CAD build for the part. Positions are in the model's coordinates, mm. A direction names the side the tool comes from. Give positions to 0.01 mm unless a question says otherwise; leave off trailing zeros. Write each loop counter-clockwise with the first axis right and the second up, starting at its lowest first coordinate (ties: lowest second). Pieces come first, ordered by that corner, then holes. Notation, with made-up numbers: (-5.75, 11.5) -> (39.25, 11.5) arc R33 ccw to (39.25, 47.5) -> close; hole circle Ø3 at (81.25, 41). An arc over 180 degrees is marked (long way). Answer as a JSON object with one key per item and string values.
```python
from build123d import *

# Parameters (mm, degrees)
SKICA2_W                 = 72.4
SKICA2_H                 = 47.7
P_IDAT_VYSUNUT_M1_DEPTH  = 1.2
SKICA3_W                 = 70
SKICA3_H                 = 46.5
P_IDAT_VYSUNUT_M2_DEPTH  = 1
SKICA4_W                 = 70
SKICA4_H                 = 7
P_IDAT_VYSUNUT_M3_DEPTH  = 7
ZKOSEN_2_SIZE            = 7
SKICA5_W                 = 15
SKICA5_H                 = 2
ODEBRAT_VYSUNUT_M1_DEPTH = 10
SKICA6_W                 = 15
SKICA6_H                 = 1.2
ODEBRAT_VYSUNUT_M2_DEPTH = 1


with BuildPart() as part:
    # Skica2 → Přidat vysunutím1 (new body)
    with BuildSketch(Plane(origin=(0, 0, 0), x_dir=(1, 0, 0), z_dir=(0, 1, 0))):
        with Locations((36.2, 23.85)):
            Rectangle(SKICA2_W, SKICA2_H)
    extrude(amount=P_IDAT_VYSUNUT_M1_DEPTH)

    # Skica3 → Přidat vysunutím2 (add)
    with BuildSketch(Plane(origin=(0, 1.2, 0), x_dir=(1, 0, 0), z_dir=(0, 1, 0))):
        with Locations((36.2, 24.45)):
            Rectangle(SKICA3_W, SKICA3_H)
    extrude(amount=P_IDAT_VYSUNUT_M2_DEPTH)

    # Skica4 → Přidat vysunutím3 (add)
    with BuildSketch(Plane(origin=(0, 2.2, 0), x_dir=(1, 0, 0), z_dir=(0, 1, 0))):
        with Locations((36.2, 44.2)):
            Rectangle(SKICA4_W, SKICA4_H)
    extrude(amount=P_IDAT_VYSUNUT_M3_DEPTH)

    # Zkosení2
    zkosen_2_edges = [part.edges().sort_by_distance(p)[0] for p in [
        (36.2, 9.2, -40.7),
    ]]
    chamfer(zkosen_2_edges, length=ZKOSEN_2_SIZE - 0.0001)  # a hair under: the kernel refuses the full size

    # Skica5 → Odebrat vysunutím1 (cut)
    with BuildSketch(Plane(origin=(0, 2.2, 0), x_dir=(1, 0, 0), z_dir=(0, 1, 0))):
        with Locations((36.2, 1)):
            Rectangle(SKICA5_W, SKICA5_H)
    extrude(amount=-ODEBRAT_VYSUNUT_M1_DEPTH, mode=Mode.SUBTRACT)

    # Skica6 → Odebrat vysunutím2 (cut)
    with BuildSketch(Plane(origin=(0, 2.2, 0), x_dir=(1, 0, 0), z_dir=(0, 1, 0))):
        with Locations((36.2, 2.6)):
            Rectangle(SKICA6_W, SKICA6_H)
    extrude(amount=-ODEBRAT_VYSUNUT_M2_DEPTH, mode=Mode.SUBTRACT)


solid = part.part
```
1) Pin check, flat tips, straight feed: pin 1 (0.5 mm diameter, centred on x = 13.5, y = 1.5, fed in from +Z); pin 2 (12 mm diameter, centred on x = 11, z = -35, fed in from +Y); pin 3 (1.1 mm diameter, centred on x = 39, y = 1.5, fed in from +Z); pin 4 (4 mm diameter, centred on y = 5, z = -21.5, fed in from -X). Stop position of each tip, or through.
Model answer:
{"pin 1": "stops at z = -1.2", "pin 2": "stops at y = 2.5", "pin 3": "stops at z = -2", "pin 4": "passes through"}
2) Mould opens along X. For faces 4 (the flat face through (28.7, 1.1, -1.6)), 5 (the flat face through (1.2, 2, -31)), 6 (the flat face through (0.5, 1.2, -13.4)) say: released by +X, released by -X, zero draft, split by the parting line, or undercut.
Model answer:
{"face 4": "undercut", "face 5": "released by -X", "face 6": "zero draft"}
3) Wall check: probe 1 along Y at (x, z) = (8.5, -16); probe 2 along X at (y, z) = (5.75, -45); probe 3 along Z at (x, y) = (50, 1.5). Give the ranges that are in metal, low to high.
Model answer:
{"probe 1": "y = 0 to 2.2", "probe 2": "x = 1.2 to 71.2", "probe 3": "z = -47.7 to -1.2"}
4) Slice it at B-B (z = -8). List the corners of the cut face in (x, y).
Model answer:
{"outline": "(0, 0) -> (72.4, 0) -> (72.4, 1.2) -> (71.2, 1.2) -> (71.2, 2.2) -> (1.2, 2.2) -> (1.2, 1.2) -> (0, 1.2) -> close"}
5) 3-axis set-ups, long thin cutter, end or side, ignore diameter. For faces 1 (the flat face through (71.2, 2, -31)), 2 (the flat face through (36, 2.2, -21)), 3 (the flat face through (43.7, 1.1, -1.6)): which of +Z, -Z, +X, -X, +Y, -Y reach the whole face in a straight line?
Model answer:
{"face 1": "+Z, -Z, +X, +Y", "face 2": "+Z, +X, -X, +Y", "face 3": "+Z, +Y"}
6) Slice it at D-D (y = 6.75). List the corners of the cut face in (x, z), then the cut area to 3 significant figures.
Model answer:
{"outline": "(1.2, -47.7) -> (71.2, -47.7) -> (71.2, -45.25) -> (1.2, -45.25) -> close", "area": "172 mm2"}
